Design review of the part built by this model. Coordinates are the model's own, in mm. Face numbers are marked on the shaded views. A direction names the side the tool comes from. Coordinates: 2 decimals unless noted, no trailing zeros. Order: outer loops, then holes, each group sorted by start corner. A loop starts at its lowest first (then second) coordinate and runs counter-clockwise, first axis right, second up. Notation, with made-up numbers: M 72.5,54 L 96.5,54 A14 ccw 96.5,64 Z; hole C -25.75,51 d2. An arc over 180 degrees is marked long. Use CSV: the item, a comma, the result in double quotes.
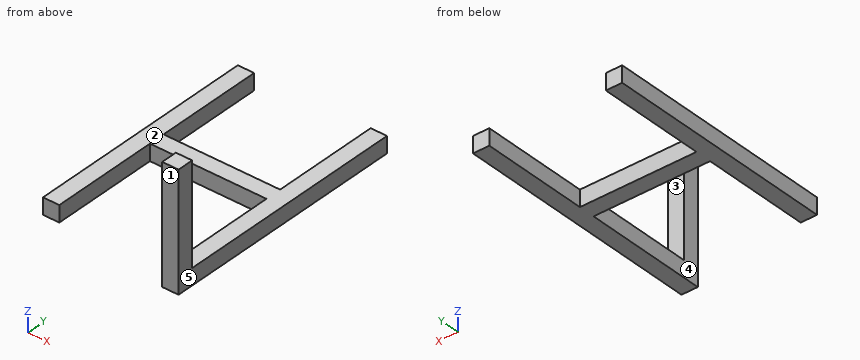
```python
from build123d import *

# Parameters (mm, degrees)
F0_W     = 70
F0_H     = 70
F1_DEPTH = 1000
F3_DEPTH = 500
F4_W     = 70
F4_H     = 70
F5_DEPTH = 535
F6_W     = 70
F6_H     = 70
F7_DEPTH = 465
F8_W     = 70
F8_H     = 70
F9_DEPTH = 500


with BuildPart() as f1:
    # F0 (on Front) → F1 (new body)
    with BuildSketch(Plane.XZ):
        Rectangle(F0_W, F0_H)
    extrude(amount=F1_DEPTH)

    # F2 (on face) → F3 (join)
    with BuildSketch(Plane.YZ.offset(35)):
        Polygon((-465, 35), (-500, 35), (-535, 35), (-535, -35), (-465, -35), align=None)
    extrude(amount=F3_DEPTH)

    # F4 (on face) → F5 (join)
    with BuildSketch(Plane.XZ.offset(535)):
        with Locations((570, 0)):
            Rectangle(F4_W, F4_H)
    extrude(amount=-F5_DEPTH)

    # F6 (on face) → F7 (join)
    with BuildSketch(Plane.XZ.offset(535)):
        with Locations((570, 0)):
            Rectangle(F6_W, F6_H)
    extrude(amount=F7_DEPTH)

    # F8 (on face) → F9 (join)
    with BuildSketch(Plane(origin=(0, 0, -35), x_dir=(1, 0, 0), z_dir=(0, 0, -1))):
        with Locations((570, 1035)):
            Rectangle(F8_W, F8_H)
    extrude(amount=-F9_DEPTH)


solid = f1.part
```
(1) Add section C-C on z = 48. State the section outline as (x, y) points, and give its area (3 significant figures).
The answers:
outline,"M 535,-1070 L 605,-1070 L 605,-1000 L 535,-1000 Z"
area,"4,900 mm2"
(2) For the marked faces 1 and 2, list the 3-axis set-ups (+Z, -Z, +X, -X, +Y, -Y) from which the entire face can be reached by the end or side of a thin tool; tool diameter is ignored.
The answers:
face 1,"+Z, -Z, +X, -X, -Y"
face 2,"+Z, +X, -X, +Y"
(3) Clearance check with flat-ended pins moving along their axes: P1, Ø21, axis at x = 338, z = 13.5, coming from the -Y side; P2, Ø1.5, axis at x = 540.5, y = -162, coming from the +Z side. State where each tip first meets the part, or that it passes through.
The answers:
P1,"stops at y = -535"
P2,"stops at z = 35"
(4) Add section A-A on y = -911. State the section outline as (x, z) points, and give its area (3 significant figures).
The answers:
outline,"M -35,-35 L 35,-35 L 35,35 L -35,35 Z; M 535,-35 L 605,-35 L 605,35 L 535,35 Z"
area,"9,800 mm2"
(5) Add section B-B on x = 48. State the section outline as (y, z) points.
The answers:
outline,"M -535,-35 L -465,-35 L -465,35 L -535,35 Z"
(6) The part is to be moulded in two halves that separate along X. For the marked faces 3, 4 and 5, say which applies: pulls with the +X half, pulls with the -X half, needs draft (parallel to the pull), parting line crosses it, or undercut.
The answers:
face 3,"needs draft"
face 4,"undercut"
face 5,"pulls with the +X half"
(7) Wall thickness on probe 1 along Y at (x, z) = (65, 19.5); probe 2 along X at (y, z) = (-168.5, 5); probe 3 along X at (y, z) = (-1023, 102): over which ranges is each line inside the solid? List them lowest first.
The answers:
probe 1,"y = -535 to -465"
probe 2,"x = -35 to 35, 535 to 605"
probe 3,"x = 535 to 605"
